Can you work these out from the drawing? Everything is in mm from the part's minimum corner. A direction names the side the tool comes from. Round coordinates to 2 decimals unless told otherwise and drop trailing zeros. Write each loop counter-clockwise with the first axis right and the second up, starting at its lowest first coordinate (ties: lowest second). Pieces come first, ordered by that corner, then holes. Notation, with made-up numbers: (8.25, -38.5) - (21.25, -38.5) arc R38 cw to (21.25, -0.5) - close; hole circle Ø6 at (19.5, 45). An arc over 180 degrees is marked (long way). One line per item, written item: value. Start each with the question number.
Item 1: For P1, Ø1.4, axis at x = 25, z = 1.5, coming from the -Y side, with a flat end and sliding along its axis, tell me the tip position at first contact or that it passes through.
Item 2: Imagine slicing it at B-B, the plane y = 26. Please give me the cut outline in (x, z).
Item 3: For the marked faces 1 and 2, which set-ups out of +Z, -Z, +X, -X, +Y, -Y let a thin tool reach every point of the face, with its end or its side?
Item 4: If I drill on line 1 (Y direction, x = 35, z = 0.6); line 2 (X direction, y = 4, z = 0.2), over which ranges is the centre line in solid material (lowest first)?
Item 5: Thinking about a two-plate mould opening in Y: for the marked faces 3, 4 and 5, which applies, released by +Y, released by -Y, zero draft, split by the parting line, or undercut?
Item 6: Imagine slicing it at C-C, the plane z = 4.2. Please give me the cut outline in (x, y), then the cut area to 3 significant figures.
Item 7: Imagine slicing it at A-A, the plane x = 18.5. Please give me the cut outline in (y, z), then the cut area to 3 significant figures.
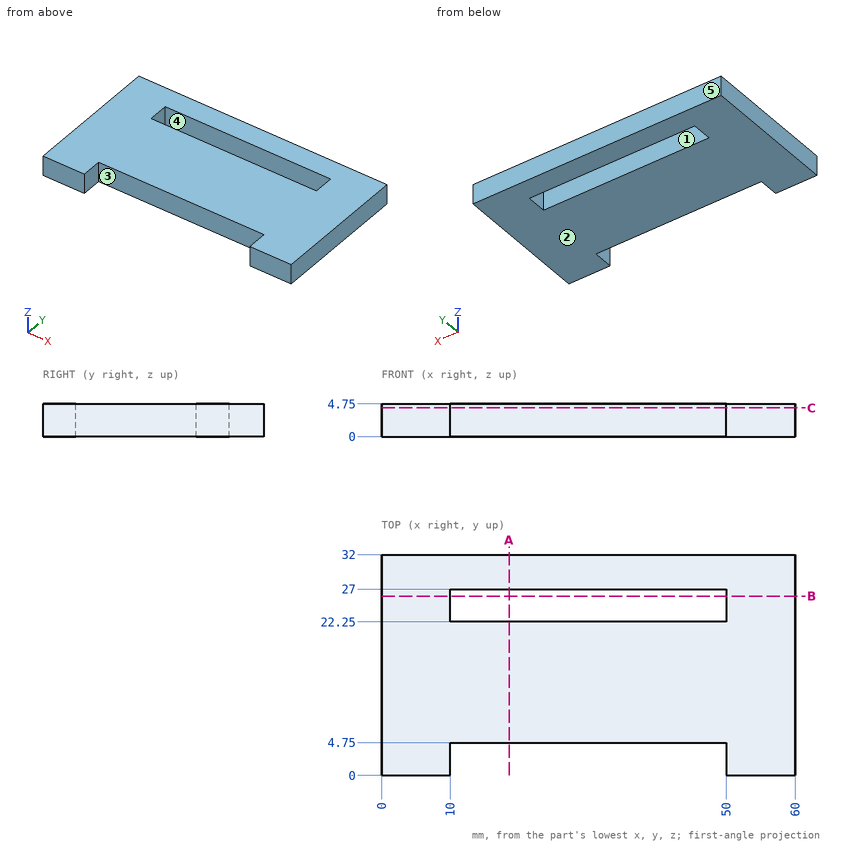
Values follow:
1. P1: stops at y = 4.75
2. outline: (0, 0) - (10, 0) - (10, 4.75) - (0, 4.75) - close; (50, 0) - (60, 0) - (60, 4.75) - (50, 4.75) - close
3. face 1: +Z, -Z
3. face 2: -Z, +X, -X, +Y, -Y
4. line 1: y = 4.75 to 22.25, 27 to 32
4. line 2: x = 0 to 10, 50 to 60
5. face 3: released by -Y
5. face 4: undercut
5. face 5: released by +Y
6. outline: (0, 0) - (10, 0) - (10, 4.75) - (50, 4.75) - (50, 0) - (60, 0) - (60, 32) - (0, 32) - close; hole (10, 22.25) - (50, 22.25) - (50, 27) - (10, 27) - close
6. area: 1,540 mm^2
7. outline: (4.75, 0) - (22.25, 0) - (22.25, 4.75) - (4.75, 4.75) - close; (27, 0) - (32, 0) - (32, 4.75) - (27, 4.75) - close
7. area: 107 mm^2
